Build history of the part. All positions in model axes, mm. Coordinates: 2 decimals unless noted, no trailing zeros. Order: outer loops, then holes, each group sorted by start corner. A loop starts at its lowest first (then second) coordinate and runs counter-clockwise, first axis right, second up. Notation, with made-up numbers: M 88,18.25 L 144,18.25 A30 cw 144,57.25 Z; hole C -5,-2.75 d11. An arc over 180 degrees is marked long. Use a Markdown table: item, result. Add a question column.
from build123d import *

# Parameters (mm, degrees)
BOSS_EXTRUDE1_DEPTH = 2
BOSS_EXTRUDE2_START = 1.5
SKETCH2_R           = 3.5
BOSS_EXTRUDE2_DEPTH = 1.5
SKETCH3_R           = 1.75
CUT_EXTRUDE1_DEPTH  = 5
SKETCH4_R           = 0.5
CUT_EXTRUDE2_DEPTH  = 5


with BuildPart() as part:
    # Sketch1 → Boss-Extrude1 (new body)
    with BuildSketch(Plane(origin=(0, 0, 0), x_dir=(1, 0, 0), z_dir=(0, 1, 0))):
        with BuildLine():
            Line((1.802775638, 3), (14.656073705, 1.99390095))
            ThreePointArc((14.656073705, 1.99390095), (16.5, 0), (14.656073705, -1.99390095))
            Line((14.656073705, -1.99390095), (1.802775638, -3))
            ThreePointArc((1.802775638, -3), (-3.5, 0), (1.802775638, 3))
        make_face()
    extrude(amount=BOSS_EXTRUDE1_DEPTH)

    # Sketch2 → Boss-Extrude2 (add)
    with BuildSketch(Plane.XZ.offset(BOSS_EXTRUDE2_START)):
        with Locations(Location((0, 0, 0), (0, 0, 270))):
            Circle(SKETCH2_R)
    extrude(amount=-BOSS_EXTRUDE2_DEPTH)

    # Sketch3 → Cut-Extrude1 (cut)
    with BuildSketch(Plane(origin=(0, 2, 0), x_dir=(1, 0, 0), z_dir=(0, 1, 0))):
        with Locations(Location((0, 0, 0), (0, 0, 270))):
            Circle(SKETCH3_R)
    extrude(amount=-CUT_EXTRUDE1_DEPTH, mode=Mode.SUBTRACT)

    # Sketch4 → Cut-Extrude2 (cut)
    with BuildSketch(Plane(origin=(0, 2, 0), x_dir=(1, 0, 0), z_dir=(0, 1, 0))):
        with Locations(Location((4.5, 0, 0), (0, 0, 270))):
            Circle(SKETCH4_R)
        with Locations(Location((6.5, 0, 0), (0, 0, 270))):
            Circle(SKETCH4_R)
        with Locations(Location((8.5, 0, 0), (0, 0, 270))):
            Circle(SKETCH4_R)
        with Locations(Location((10.5, 0, 0), (0, 0, 270))):
            Circle(SKETCH4_R)
        with Locations(Location((12.5, 0, 0), (0, 0, 270))):
            Circle(SKETCH4_R)
        with Locations(Location((14.5, 0, 0), (0, 0, 270))):
            Circle(SKETCH4_R)
    extrude(amount=-CUT_EXTRUDE2_DEPTH, mode=Mode.SUBTRACT)


solid = part.part
(1) Slice it at C-C on y = -0.95. Give the cut face in (x, z), and give its area (3 significant figures).
(2) Mould opens along Z. For faces 1 (the cylindrical face through (5, 1, 0)), 2 (the flat face through (9.3, 0, 0)), 3 (the cylindrical face through (16.5, 1, 0)), 4 (the cylindrical face through (12, 1, 0)) say: released by +Z, released by -Z, zero draft, split by the parting line, or undercut.
(3) Slice it at B-B on x = 8.75. Give the cut face in (y, z).
(4) Slice it at D-D on x = 6.5. Give the cut face in (y, z), and give its area (3 significant figures).
(5) Slice it at A-A on z = 1. Give the cut face in (x, y), and give its area (3 significant figures).
(6) Drill centre lines: line 1 along X through (y, z) = (-0.25, 0); line 2 along Z through (x, y) = (0.75, 1.75); line 3 along Y through (x, z) = (11, -0.25). Where is each one in solid material? Low to high. Write a range as from..to.
(7) Drop flat-ended pins along their axis: P1, Ø1.5, axis at x = 4.5, y = 0, coming from the +Z side; P2, Ø1.5, axis at x = 13, z = 1, coming from the -Y side; P3, Ø2, axis at x = 6, y = 1, coming from the -Z side. Give the stop position or say it passes through.
Solutions:
| question | item | result |
|---|---|---|
| 1 | outline | C 0,0 d7; hole C 0,0 d3.5 |
| 1 | area | 28.9 mm² |
| 2 | face 1 | undercut |
| 2 | face 2 | zero draft |
| 2 | face 3 | split by the parting line |
| 2 | face 4 | undercut |
| 3 | outline | M 0,-2.46 L 2,-2.46 L 2,-0.43 L 0,-0.43 Z; M 0,0.43 L 2,0.43 L 2,2.46 L 0,2.46 Z |
| 4 | outline | M 0,-2.63 L 2,-2.63 L 2,-0.5 L 0,-0.5 Z; M 0,0.5 L 2,0.5 L 2,2.63 L 0,2.63 Z |
| 4 | area | 8.53 mm² |
| 5 | outline | M -3.35,-1.5 L -1.44,-1.5 L -1.44,2 L -3.35,2 Z; M 1.44,-1.5 L 3.35,-1.5 L 3.35,0 L 16.23,0 L 16.23,2 L 1.44,2 Z |
| 5 | area | 39.2 mm² |
| 6 | line 1 | -3.5..-1.75, 1.75..3.5 |
| 6 | line 2 | -3.42..-1.58, 1.58..3.42 |
| 6 | line 3 | 0..2 |
| 7 | P1 | z = 2.85 |
| 7 | P2 | y = 0 |
| 7 | P3 | z = -2.75 |
